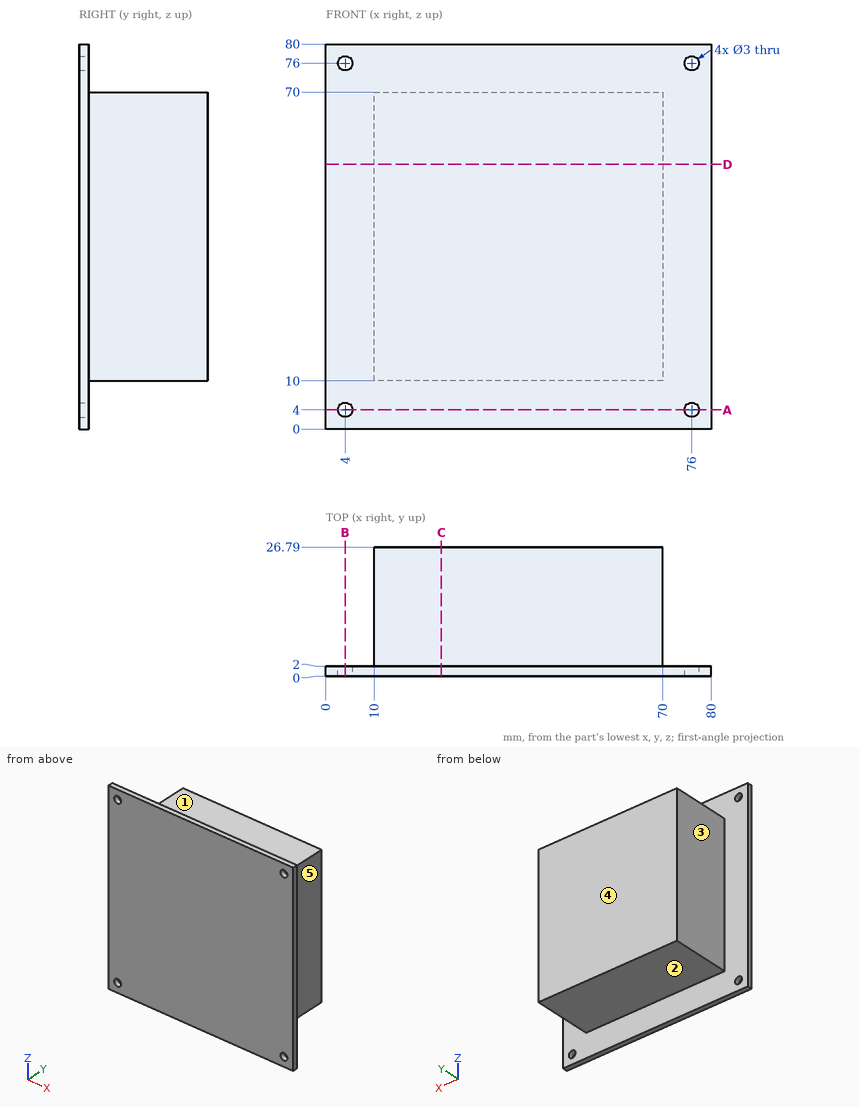
Source: three-view drawing plus pictorial views. Frame: mm from the lowest corner of the part. A direction names the side the tool comes from. Coordinates: 2 decimals unless noted, no trailing zeros. Order: outer loops, then holes, each group sorted by start corner. A loop starts at its lowest first (then second) coordinate and runs counter-clockwise, first axis right, second up. Notation, with made-up numbers: M 22,-24.75 L 64,-24.75 A33 ccw 64,11.25 Z; hole C 83,63 d5. An arc over 180 degrees is marked long. Answer in a Markdown table with one row per item.
(1) Section query B-B, the plane x = 4. Output: boundary loops of the cut face in (y, z), plus the area to 3 significant figures.
Numbers:
| item | result |
|---|---|
| outline | M 0,0 L 2,0 L 2,2.5 L 0,2.5 Z; M 0,5.5 L 2,5.5 L 2,74.5 L 0,74.5 Z; M 0,77.5 L 2,77.5 L 2,80 L 0,80 Z |
| area | 148 mm^2 |
(2) Section query D-D, the plane z = 55. Output: boundary loops of the cut face in (x, y).
Numbers:
| item | result |
|---|---|
| outline | M 0,0 L 80,0 L 80,2 L 70,2 L 70,26.79 L 10,26.79 L 10,2 L 0,2 Z |
(3) Contact query for flat-ended pins moving along their axis: pin 1 Ø2 at (x, y) = (50.5, 20) entering from -Z; pin 2 Ø4 at (x, y) = (37.5, 12) entering from +Z; pin 3 Ø4 at (y, z) = (12, 57.5) entering from +X. Output: stop coordinate, or through.
Numbers:
| item | result |
|---|---|
| pin 1 | stops at z = 10 |
| pin 2 | stops at z = 70 |
| pin 3 | stops at x = 70 |
(4) Section query A-A, the plane z = 4. Output: boundary loops of the cut face in (x, y), plus the area to 3 significant figures.
Numbers:
| item | result |
|---|---|
| outline | M 0,0 L 2.5,0 L 2.5,2 L 0,2 Z; M 5.5,0 L 74.5,0 L 74.5,2 L 5.5,2 Z; M 77.5,0 L 80,0 L 80,2 L 77.5,2 Z |
| area | 148 mm^2 |
(5) Material intervals for line 1 (X direction, y = 0.55, z = 4); line 2 (Y direction, x = 5.5, z = 23.5), sorted ascending. Write a range as [from, to].
Numbers:
| item | result |
|---|---|
| line 1 | x = [0, 2.5], [5.5, 74.5], [77.5, 80] |
| line 2 | y = [0, 2] |
(6) Access query for the marked faces 1, 2, 3, 4 and 5. Directions: +Z, -Z, +X, -X, +Y, -Y. A direction counts if a zero-diameter tool reaches every point of the face in a straight line with its end or side. Return the directions, or none.
Numbers:
| item | result |
|---|---|
| face 1 | +Z, +X, -X, +Y |
| face 2 | -Z, +X, -X, +Y |
| face 3 | +Z, -Z, -X, +Y |
| face 4 | +Z, -Z, +X, -X, +Y |
| face 5 | +Z, -Z, +X, +Y |
(7) Section query C-C, the plane x = 24. Output: boundary loops of the cut face in (y, z), plus the area to 3 significant figures.
Numbers:
| item | result |
|---|---|
| outline | M 0,0 L 2,0 L 2,10 L 26.79,10 L 26.79,70 L 2,70 L 2,80 L 0,80 Z |
| area | 1,650 mm^2 |
